```python
from build123d import *

# Parameters (mm, degrees)
SKETCH1_W           = 28
SKETCH1_H           = 5
BOSS_EXTRUDE1_DEPTH = 20
CHAMFER1_SIZE       = 15
BOSS_EXTRUDE2_DEPTH = 28
SKETCH3_W           = 3
SKETCH3_H           = 9
CUT_EXTRUDE1_DEPTH  = 12.8
CHAMFER2_SIZE       = 1
FILLET1_R           = 2
CHAMFER3_SIZE       = 0.5
CUT_EXTRUDE2_DEPTH  = 12.8
CHAMFER4_SIZE       = 3
CHAMFER5_SIZE       = 3
SKETCH8_W           = 3.20799886
SKETCH8_H           = 3.210000155
SKETCH8_W_2         = 3.209995615
SKETCH8_H_2         = 3.268000248
CUT_EXTRUDE3_DEPTH  = 5.4


with BuildPart() as part:
    # Sketch1 → Boss-Extrude1 (new body)
    with BuildSketch(Plane(origin=(0, 0, 0), x_dir=(1, 0, 0), z_dir=(0, 1, 0))):
        with Locations((14, 2.5)):
            Rectangle(SKETCH1_W, SKETCH1_H)
    extrude(amount=BOSS_EXTRUDE1_DEPTH)

    # Chamfer1
    chamfer1_edges = [part.edges().sort_by_distance(p)[0] for p in [
        (28, 0, -2.5),
    ]]
    chamfer(chamfer1_edges, length=CHAMFER1_SIZE)

    # Sketch2 → Boss-Extrude2 (add)
    with BuildSketch(Plane.XY):
        Polygon((9.648757297, 6.5), (5, 6.5), (5, 2), (5, 0), (9.648757297, 0), align=None)
    extrude(amount=BOSS_EXTRUDE2_DEPTH)

    # Sketch3 → Cut-Extrude1 (cut)
    with BuildSketch(Plane.XZ):
        with Locations((6.5, 18)):
            Rectangle(SKETCH3_W, SKETCH3_H)
    extrude(amount=-CUT_EXTRUDE1_DEPTH, mode=Mode.SUBTRACT)

    # Chamfer2
    chamfer2_edges = [part.edges().sort_by_distance(p)[0] for p in [
        (8, 3.25, 22.5),
        (8, 3.25, 13.5),
    ]]
    chamfer(chamfer2_edges, length=CHAMFER2_SIZE)

    # Fillet1
    fillet1_edges = [part.edges().sort_by_distance(p)[0] for p in [
        (7.324378649, 6.5, 28),
        (7.324378649, 0, 28),
    ]]
    fillet(fillet1_edges, radius=FILLET1_R)

    # Chamfer3
    chamfer3_edges = [part.edges().sort_by_distance(p)[0] for p in [
        (5, 3.25, 13.5),
        (5, 3.25, 22.5),
    ]]
    chamfer(chamfer3_edges, length=CHAMFER3_SIZE)

    # Sketch4 → Cut-Extrude2 (cut)
    with BuildSketch(Plane.ZY.offset(-5)):
        with BuildLine():
            ThreePointArc((25.5, 1.45), (27.05, 3), (25.5, 4.55))
            ThreePointArc((25.5, 4.55), (23.95, 3), (25.5, 1.45))
        make_face()
        with BuildLine():
            ThreePointArc((10.5, 4.55), (8.95, 3), (10.5, 1.45))
            ThreePointArc((10.5, 1.45), (12.05, 3), (10.5, 4.55))
        make_face()
    extrude(amount=-CUT_EXTRUDE2_DEPTH, mode=Mode.SUBTRACT)

    # Chamfer4
    chamfer4_edges = [part.edges().sort_by_distance(p)[0] for p in [
        (5, 3.25, 0),
        (9.648757297, 3.25, 0),
    ]]
    chamfer(chamfer4_edges, length=CHAMFER4_SIZE)

    # Chamfer5
    chamfer5_edges = [part.edges().sort_by_distance(p)[0] for p in [
        (7.324378649, 6.5, 0),
    ]]
    chamfer(chamfer5_edges, length=CHAMFER5_SIZE)

    # Sketch8 → Cut-Extrude3 (cut)
    # profile 1 of 4: a face of its own
    with BuildSketch(Plane(origin=(0, 20, 0), x_dir=(1, 0, 0), z_dir=(0, 1, 0))):
        with Locations((5.668003112, 2.226999903)):
            Rectangle(SKETCH8_W, SKETCH8_H)
        Polygon((7.122002542, 3.68199998), (6.328001618, 3.68199998), (4.214003682, 3.68199998), (4.214003682, 2.801999915), (4.214003682, 2.091999864), (4.214003682, 0.771999825), (4.858002067, 0.771999825), (6.60200417, 0.771999825), (7.122002542, 0.771999825), (7.122002542, 3.48399987), align=None, mode=Mode.SUBTRACT)
    # profile 2 of 4: a face of its own
    with BuildSketch(Plane(origin=(0, 20, 0), x_dir=(1, 0, 0), z_dir=(0, 1, 0))):
        Polygon((7.122002542, 3.68199998), (7.122002542, 3.48399987), (7.122002542, 0.771999825), (6.60200417, 0.771999825), (4.858002067, 0.771999825), (4.214003682, 0.771999825), (4.214003682, 2.091999864), (4.214003682, 2.801999915), (4.214003682, 3.68199998), (6.328001618, 3.68199998), align=None)
    # profile 3 of 4: a face of its own
    with BuildSketch(Plane(origin=(0, 20, 0), x_dir=(1, 0, 0), z_dir=(0, 1, 0))):
        with Locations((23.709002883, 2.229999751)):
            Rectangle(SKETCH8_W_2, SKETCH8_H_2)
        Polygon((22.254005075, 1.15799997), (22.254005075, 1.283999765), (22.254005075, 3.713999875), (25.16400069, 3.713999875), (25.16400069, 0.749999657), (25.16400069, 0.745999627), (24.429999292, 0.745999627), (22.254005075, 0.745999627), align=None, mode=Mode.SUBTRACT)
    # profile 4 of 4: a face of its own
    with BuildSketch(Plane(origin=(0, 20, 0), x_dir=(1, 0, 0), z_dir=(0, 1, 0))):
        Polygon((22.254005075, 3.713999875), (22.254005075, 1.283999765), (22.254005075, 1.15799997), (22.254005075, 0.745999627), (24.429999292, 0.745999627), (25.16400069, 0.745999627), (25.16400069, 0.749999657), (25.16400069, 3.713999875), align=None)
    extrude(amount=-CUT_EXTRUDE3_DEPTH, mode=Mode.SUBTRACT)


solid = part.part
```
Model file for the job. Use its own axes, mm. A direction names the side the tool comes from. Coordinates: 2 decimals unless noted, no trailing zeros. Loops run counter-clockwise (first coordinate to the right, second up) from the corner with the lowest first, then second, coordinate; pieces in that order, holes last. Notation, with made-up numbers: (-36.5, -24.5) -> (-25.5, -24.5) arc R17 ccw to (-25.5, -7.5) -> close; hole circle Ø6 at (50, 46). An arc over 180 degrees is marked (long way). Answer as a JSON object with one key per item and string values.
Q1. Cut at C-C (y = 18.5). List the corners of the cut face in (x, z), and give its area (3 significant figures).
Report:
{"outline": "(0, -5) -> (28, -5) -> (28, 0) -> (0, 0) -> close; hole (4.06, -3.83) -> (7.27, -3.83) -> (7.27, -0.62) -> (4.06, -0.62) -> close; hole (22.1, -3.86) -> (25.31, -3.86) -> (25.31, -0.6) -> (22.1, -0.6) -> close", "area": "119 mm2"}
Q2. Cut at A-A (z = 25.5). List the corners of the cut face in (x, y).
Report:
{"outline": "(5, 0) -> (9.65, 0) -> (9.65, 1.45) -> (5, 1.45) -> close; (5, 4.55) -> (9.65, 4.55) -> (9.65, 6.5) -> (5, 6.5) -> close"}
Q3. Cut at D-D (z = 11). List the corners of the cut face in (x, y).
Report:
{"outline": "(5, 0) -> (9.65, 0) -> (9.65, 1.53) -> (5, 1.53) -> close; (5, 4.47) -> (9.65, 4.47) -> (9.65, 6.5) -> (5, 6.5) -> close"}
Q4. Cut at B-B (y = 3). List the corners of the cut face in (x, z).
Report:
{"outline": "(0, -5) -> (16, -5) -> (16, 0) -> (12.65, 0) -> (9.65, 3) -> (9.65, 8.95) -> (5, 8.95) -> (5, 3) -> (2, 0) -> (0, 0) -> close; (5, 12.05) -> (9.65, 12.05) -> (9.65, 23.95) -> (5, 23.95) -> (5, 23) -> (5.5, 22.5) -> (7, 22.5) -> (8, 21.5) -> (8, 14.5) -> (7, 13.5) -> (5.5, 13.5) -> (5, 13) -> close; (5, 27.05) -> (9.65, 27.05) -> (9.65, 28) -> (5, 28) -> close"}
Q5. 3-axis set-ups, long thin cutter, end or side, ignore diameter. For faces 1 (the flat face through (7.5, 3.2, 14)), 2 (the flat face through (9.649, 3, 15)), 3 (the flat face through (22.104, 17, -2)): which of +Z, -Z, +X, -X, +Y, -Y reach the whole face in a straight line?
Report:
{"face 1": "-X, +Y, -Y", "face 2": "+Z, +X, +Y, -Y", "face 3": "+Y"}
Q6. Flat gauge pins, fed straight in: P1, Ø5, axis at y = 4.5, z = 10, coming from the -X side; P2, Ø2.5, axis at x = 24, z = -2, coming from the +Y side; P3, Ø10, axis at x = 20.5, y = 12, coming from the +Z side; P4, Ø2.5, axis at y = 3, z = 10.5, coming from the +X side. Where does each tip first touch, or does it go through?
Report:
{"P1": "stops at x = 5", "P2": "stops at y = 14.6", "P3": "stops at z = 0", "P4": "passes through"}
Q7. Probe probe 1 along X at (y, z) = (19.25, -2); probe 2 along Z at (x, y) = (8.5, 3); probe 3 along Y at (x, z) = (7.65, 25.5). List the from-to ranges inside material, lowest first.
Report:
{"probe 1": "x = 0 to 4.06, 7.27 to 22.1, 25.31 to 28", "probe 2": "z = -5 to 8.95, 12.05 to 23.95, 27.05 to 28", "probe 3": "y = 0 to 1.45, 4.55 to 6.5"}
Q8. Pull direction X, two halves, no side cores. Call faces 4 (the flat face through (6, 14.6, -2)), 5 (the cylindrical face through (7.29, 5.9, 27.43)), 6 (the flat face through (5, 3, 8)), 7 (the flat face through (24, 14.6, -2)): released by +X, released by -X, zero draft, split by the parting line, or undercut.
Report:
{"face 4": "undercut", "face 5": "zero draft", "face 6": "released by -X", "face 7": "undercut"}
